Geometry check sheet. Reference: the model listing, model coordinates, mm. Face numbers are marked on the shaded views. A direction names the side the tool comes from. Round coordinates to 2 decimals unless told otherwise and drop trailing zeros. Loops run counter-clockwise (first coordinate to the right, second up) from the corner with the lowest first, then second, coordinate; pieces in that order, holes last.
```python
from build123d import *

# Parameters (mm, degrees)
EXTRUDE_1_DEPTH     = 10
SKETCH_3_R          = 1.6
CUT_EXTRUDE_1_DEPTH = 10


with BuildPart() as part:
    # 草图2 → 凸台-拉伸1 (new body)
    with BuildSketch(Plane(origin=(0, 0, 0), x_dir=(0, 0, -1), z_dir=(1, 0, 0))):
        with BuildLine():
            Line((-12.649110641, 6), (-20, 6))
            Line((-20, 6), (-20, 8))
            Line((-20, 8), (-13.856406461, 8))
            ThreePointArc((-13.856406461, 8), (0, 16), (13.856406461, 8))
            Line((13.856406461, 8), (20, 8))
            Line((20, 8), (20, 6))
            Line((20, 6), (12.649110641, 6))
            ThreePointArc((12.649110641, 6), (0, 14), (-12.649110641, 6))
        make_face()
    extrude(amount=EXTRUDE_1_DEPTH)

    # 草图3 → 切除-拉伸1 (cut)
    with BuildSketch(Plane(origin=(0, 8, 0), x_dir=(1, 0, 0), z_dir=(0, 1, 0))):
        with Locations(Location((5, 16.785, 0), (0, 0, 270))):
            Circle(SKETCH_3_R)
        with Locations(Location((5, -16.785, 0), (0, 0, 270))):
            Circle(SKETCH_3_R)
    extrude(amount=-CUT_EXTRUDE_1_DEPTH, mode=Mode.SUBTRACT)


solid = part.part
```
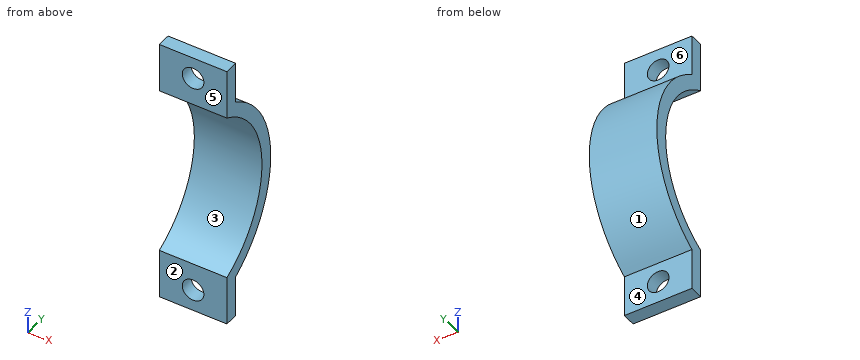
1) Sectioned sample at B-B, the plane y = 9.75. Record the cut outline in (x, z).
Report:
outline: (0, -12.69) - (10, -12.69) - (10, -10.05) - (0, -10.05) - close; (0, 10.05) - (10, 10.05) - (10, 12.69) - (0, 12.69) - close
2) Gauge pin test, flat ends, axial feed: pin 1 (3 mm diameter, centred on x = 4, z = -18.5, fed in from +Y); pin 2 (4 mm diameter, centred on x = 8.5, y = 12.5, fed in from -Z); pin 3 (2 mm diameter, centred on x = 8, z = -4.5, fed in from -Y). Record the tip position at first contact, or that the pin passes through.
Report:
pin 1: stops at y = 8
pin 2: stops at z = -12.07
pin 3: stops at y = 12.87
3) Sectioned sample at C-C, the plane x = 7.75. Record the cut outline in (y, z).
Report:
outline: (6, -20) - (8, -20) - (8, -13.86) arc R16 ccw to (8, 13.86) - (8, 20) - (6, 20) - (6, 12.65) arc R14 cw to (6, -12.65) - close
4) Scan lines: line 1 along Z through (x, y) = (3.5, 9); line 2 along Y through (x, z) = (6.25, -14); line 3 along X through (y, z) = (7.75, 16.5). Record each from-to range of solid material in increasing order.
Report:
line 1: z = -13.23 to -10.72, 10.72 to 13.23
line 2: y = 6 to 8
line 3: x = 0 to 3.43, 6.57 to 10
5) Sectioned sample at D-D, the plane z = -6. Record the cut outline in (x, y), then the cut area to 3 significant figures.
Report:
outline: (0, 12.65) - (10, 12.65) - (10, 14.83) - (0, 14.83) - close
area: 21.8 mm2
6) Access from +Z, -Z, +X, -X, +Y, -Y to the whole of each face (thin tool, end or side, straight path). Record for the marked faces 4, 5 and 6.
Report:
face 4: -Z, +X, -X, +Y
face 5: +Z, -Z, +X, -X, -Y
face 6: +Z, +X, -X, +Y
7) Sectioned sample at A-A, the plane x = 5. Record the cut outline in (y, z) (3 decimals), then the cut area to 3 significant figures.
Report:
outline: (6, -20) - (8, -20) - (8, -18.385) - (6, -18.385) - close; (6, -15.185) - (8, -15.185) - (8, -13.856) arc R16 ccw to (8, 13.856) - (8, 15.185) - (6, 15.185) - (6, 12.649) arc R14 cw to (6, -12.649) - close; (6, 18.385) - (8, 18.385) - (8, 20) - (6, 20) - close
area: 79.3 mm2
8) Mould release check, pull along Z, two halves, no side actions. Record for the marked faces 1, 2 and 3: +Z half, -Z half, draft (parallel to the pull), parting line (faces both ways), or undercut.
Report:
face 1: parting line
face 2: draft
face 3: undercut
